```python
from build123d import *

# Parameters (mm, degrees)
SKETCH2_R           = 2.0828
SKETCH2_R_2         = 20.32
BOSS_EXTRUDE1_DEPTH = 6.35


with BuildPart() as part:
    # Sketch2 → Boss-Extrude1 (new body)
    with BuildSketch(Plane(origin=(0, 0, 0), x_dir=(1, 0, 0), z_dir=(0, 1, 0))):
        Polygon((15.875, 0), (15.875, 12.7), (9.525, 12.7), (9.525, 25.4), (15.875, 25.4), (15.875, 38.1), (9.525, 38.1), (9.525, 50.8), (15.875, 50.8), (15.875, 63.5), (9.525, 63.5), (9.525, 76.2), (15.875, 76.2), (15.875, 88.9), (9.525, 88.9), (9.525, 101.6), (15.875, 101.6), (15.875, 114.3), (9.525, 114.3), (9.525, 127), (15.875, 127), (193.675, 127), (193.675, 114.3), (200.025, 114.3), (200.025, 101.6), (193.675, 101.6), (193.675, 88.9), (200.025, 88.9), (200.025, 76.2), (193.675, 76.2), (193.675, 63.5), (200.025, 63.5), (200.025, 50.8), (193.675, 50.8), (193.675, 38.1), (200.025, 38.1), (200.025, 25.4), (193.675, 25.4), (193.675, 12.7), (200.025, 12.7), (200.025, 0), align=None)
        with Locations(Location((41.275, 57.15, 0), (0, 0, 270))):
            Circle(SKETCH2_R, mode=Mode.SUBTRACT)
        with Locations(Location((168.275, 57.15, 0), (0, 0, 90))):
            Circle(SKETCH2_R, mode=Mode.SUBTRACT)
        with Locations(Location((130.175, 29.972, 0), (0, 0, 270))):
            Circle(SKETCH2_R_2, mode=Mode.SUBTRACT)
        with Locations(Location((22.225, 6.35, 0), (0, 0, 270))):
            Circle(SKETCH2_R, mode=Mode.SUBTRACT)
        with Locations(Location((187.325, 6.35, 0), (0, 0, 90))):
            Circle(SKETCH2_R, mode=Mode.SUBTRACT)
    extrude(amount=BOSS_EXTRUDE1_DEPTH)


solid = part.part
```
CAD build for the part. Positions are in the model's coordinates, mm. A direction names the side the tool comes from. Round coordinates to 2 decimals unless told otherwise and drop trailing zeros. Loops run counter-clockwise (first coordinate to the right, second up) from the corner with the lowest first, then second, coordinate; pieces in that order, holes last. Notation, with made-up numbers: M 13,-24.75 L 48,-24.75 A15 cw 48,-14.75 Z; hole C 18.5,67 d6. An arc over 180 degrees is marked long. Use a Markdown table: item, result. Add a question column.
(1) Drill centre lines: line 1 (X direction, y = 3.25, z = -57) (3 decimals); line 2 (Z direction, x = 168, y = 1.5); line 3 (X direction, y = 5.75, z = -5) (3 decimals). Where is each one in solid material? Low to high.
(2) Which spindle directions (+Z, -Z, +X, -X, +Y, -Y) get a long thin tool onto all of the face, cutting with end or side? Do faces 1 (the face through (15.875, 3, -82)), 2 (the face through (193.675, 3, -121)), 3 (the face through (197, 3, -25.4)). Say none if no direction does.
(3) Cut at C-C (z = -34). Give the cut face in (x, y) (3 decimals).
(4) Pull direction X, two halves, no side cores. Call faces 4 (the face through (200.025, 3, -32)), 5 (the face through (197, 3, -38.1)), 6 (the face through (185.26, 3.13, -6.08)), 7 (the face through (170.31, 3.13, -56.7)): +X half, -X half, draft (parallel to the pull), parting line (faces both ways), or undercut.
(5) Cut at B-B (x = 148). Give the cut face in (y, z).
(6) Flat gauge pins, fed straight in: pin 1 (3 mm diameter, centred on x = 47, y = 3.5, fed in from +Z); pin 2 (1.9 mm diameter, centred on x = 11, y = 2.5, fed in from +Z); pin 3 (3 mm diameter, centred on y = 3.5, z = -68, fed in from +X) (3 decimals); pin 4 (3 mm diameter, centred on y = 2.5, z = -54.5, fed in from -X) (3 decimals). Where does each tip first touch, or does it go through?
(7) Cut at D-D (z = -61.5). Give the cut face in (x, y) (3 decimals), and give its area (3 significant figures).
(8) Cut at A-A (z = -6.35). Give the cut face in (x, y) (3 decimals).
Geometry says:
| question | item | result |
|---|---|---|
| 1 | line 1 | x = 15.875 to 39.198, 43.352 to 166.198, 170.352 to 200.025 |
| 1 | line 2 | z = -127 to -59.21, -55.09 to 0 |
| 1 | line 3 | x = 15.875 to 20.639, 23.811 to 185.739, 188.911 to 200.025 |
| 2 | face 1 | -X, +Y, -Y |
| 2 | face 2 | -Z, +X, +Y, -Y |
| 2 | face 3 | +X, +Y, -Y |
| 3 | outline | M 15.875,0 L 110.258,0 L 110.258,6.35 L 15.875,6.35 Z; M 150.092,0 L 200.025,0 L 200.025,6.35 L 150.092,6.35 Z |
| 4 | face 4 | +X half |
| 4 | face 5 | draft |
| 4 | face 6 | undercut |
| 4 | face 7 | undercut |
| 5 | outline | M 0,-127 L 6.35,-127 L 6.35,-39.73 L 0,-39.73 Z; M 0,-20.22 L 6.35,-20.22 L 6.35,0 L 0,0 Z |
| 6 | pin 1 | stops at z = 0 |
| 6 | pin 2 | stops at z = -12.7 |
| 6 | pin 3 | stops at x = 193.675 |
| 6 | pin 4 | stops at x = 15.875 |
| 7 | outline | M 15.875,0 L 200.025,0 L 200.025,6.35 L 15.875,6.35 Z |
| 7 | area | 1,170 mm² |
| 8 | outline | M 15.875,0 L 20.142,0 L 20.142,6.35 L 15.875,6.35 Z; M 24.308,0 L 185.242,0 L 185.242,6.35 L 24.308,6.35 Z; M 189.408,0 L 200.025,0 L 200.025,6.35 L 189.408,6.35 Z |
